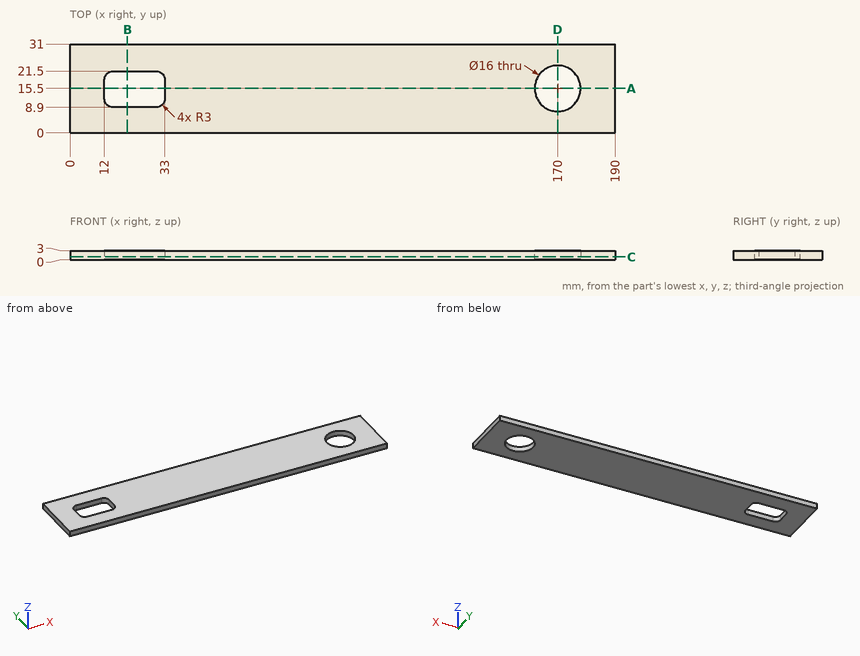
Could you check a few things on this drawing? It's one solid part, dimensions in mm from its lowest x, y, z. Coordinates: 2 decimals unless noted, no trailing zeros. Order: outer loops, then holes, each group sorted by start corner. A loop starts at its lowest first (then second) coordinate and runs counter-clockwise, first axis right, second up.
1. If we section it at B-B (x = 20): Please give me the cut outline in (y, z), then the cut area to 3 significant figures.
2. I'm going to push a flat-ended pin straight in: pin 1 (1 mm diameter, centred on x = 146, y = 8.5, fed in from -Z). Where does the tip first touch, or does it pass through?
3. If we section it at C-C (z = 0.9): Please give me the cut outline in (x, y).
4. I need wall thicknesses on line 1 (Y direction, x = 170, z = 1.25); line 2 (X direction, y = 9.5, z = 1.3); line 3 (Y direction, x = 19, z = 0.4). Which ranges of each line are inside material? Lowest first, please.
5. If we section it at D-D (x = 170): Please give me the cut outline in (y, z), then the cut area to 3 significant figures.
6. If we section it at A-A (y = 15.5): Please give me the cut outline in (x, z).
Entries:
1. outline: (0, 0) - (8.9, 0) - (8.9, 3) - (0, 3) - close; (21.5, 0) - (31, 0) - (31, 3) - (21.5, 3) - close
1. area: 55.2 mm2
2. pin 1: stops at z = 0
3. outline: (0, 0) - (190, 0) - (190, 31) - (0, 31) - close; hole (12, 11.9) arc R3 ccw to (15, 8.9) - (30, 8.9) arc R3 ccw to (33, 11.9) - (33, 18.5) arc R3 ccw to (30, 21.5) - (15, 21.5) arc R3 ccw to (12, 18.5) - close; hole circle Ø16 at (170, 15.5)
4. line 1: y = 0 to 7.5, 23.5 to 31
4. line 2: x = 0 to 13.2, 31.8 to 164.71, 175.29 to 190
4. line 3: y = 0 to 8.9, 21.5 to 31
5. outline: (0, 0) - (7.5, 0) - (7.5, 3) - (0, 3) - close; (23.5, 0) - (31, 0) - (31, 3) - (23.5, 3) - close
5. area: 45.0 mm2
6. outline: (0, 0) - (12, 0) - (12, 3) - (0, 3) - close; (33, 0) - (162, 0) - (162, 3) - (33, 3) - close; (178, 0) - (190, 0) - (190, 3) - (178, 3) - close
